The figure shows three views and two pictorial views of one solid part (mm, origin at its lowest corner). Answer the questions. A direction names the side the tool comes from. Coordinates: 2 decimals unless noted, no trailing zeros. Order: outer loops, then holes, each group sorted by start corner. A loop starts at its lowest first (then second) coordinate and runs counter-clockwise, first axis right, second up. Notation, with made-up numbers: M -26,66 L 24,66 A18 ccw 24,73 Z; hole C 9.5,48 d6. An arc over 180 degrees is marked long. Use a Markdown table: item, result.
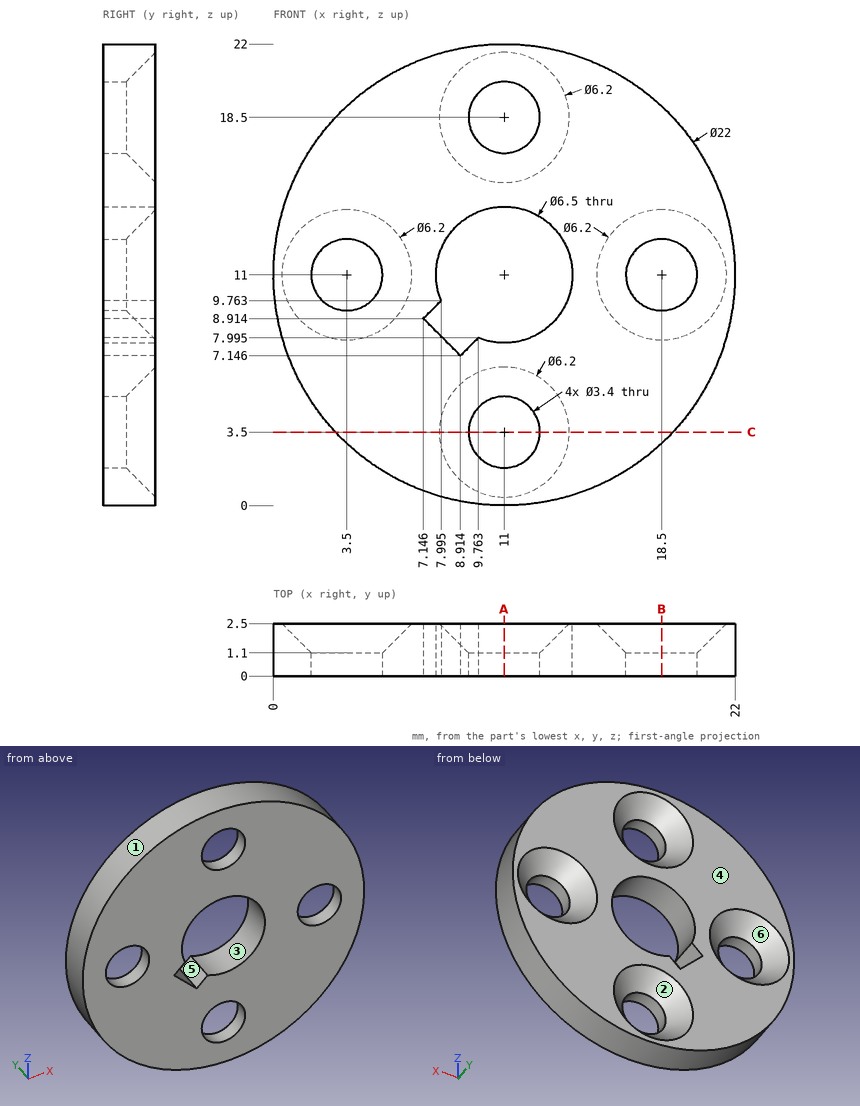
1. Section C-C on z = 3.5 is taken. Determine the outline of the cut face in (x, y).
Answers below:
| item | result |
|---|---|
| outline | M 2.95,0 L 9.3,0 L 9.3,1.1 L 7.9,2.5 L 2.95,2.5 Z; M 12.7,0 L 19.05,0 L 19.05,2.5 L 14.1,2.5 L 12.7,1.1 Z |
2. For a pull along Z with two mould halves and no side action, classify the marked faces 1, 2, 3 and 4 as +Z half, -Z half, draft (parallel to the pull), parting line (faces both ways), or undercut.
Answers below:
| item | result |
|---|---|
| face 1 | parting line |
| face 2 | undercut |
| face 3 | undercut |
| face 4 | draft |
3. Section B-B on x = 18.5 is taken. Determine the outline of the cut face in (y, z).
Answers below:
| item | result |
|---|---|
| outline | M 0,2.95 L 2.5,2.95 L 2.5,7.9 L 1.1,9.3 L 0,9.3 Z; M 0,12.7 L 1.1,12.7 L 2.5,14.1 L 2.5,19.05 L 0,19.05 Z |
4. Flat-ended cylindrical pins translate along their axes: P1, Ø4, axis at x = 11, z = 3.5, coming from the +Y side; P2, Ø2.5, axis at x = 18.5, z = 11, coming from the +Y side. Find the tip coordinate at first contact, or state that the pin passes through.
Answers below:
| item | result |
|---|---|
| P1 | y = 1.4 |
| P2 | through |
5. Find the intervals of material crossed by probe 1 along X at (y, z) = (0.7, 11); probe 2 along X at (y, z) = (1.6, 11.5) (1 decimal); probe 3 along Z at (x, y) = (8.75, 1.95) (1 decimal), in increasing order.
Answers below:
| item | result |
|---|---|
| probe 1 | 0 to 1.8, 5.2 to 7.75, 14.25 to 16.8, 20.2 to 22 |
| probe 2 | 0 to 1.4, 5.6 to 7.8, 14.2 to 16.4, 20.6 to 22 |
| probe 3 | 0.2 to 2.3, 4.7 to 7.3, 13.3 to 17.3, 19.7 to 21.8 |
6. Section A-A on x = 11 is taken. Determine the outline of the cut face in (y, z).
Answers below:
| item | result |
|---|---|
| outline | M 0,0 L 2.5,0 L 2.5,0.4 L 1.1,1.8 L 0,1.8 Z; M 0,5.2 L 1.1,5.2 L 2.5,6.6 L 2.5,7.75 L 0,7.75 Z; M 0,14.25 L 2.5,14.25 L 2.5,15.4 L 1.1,16.8 L 0,16.8 Z; M 0,20.2 L 1.1,20.2 L 2.5,21.6 L 2.5,22 L 0,22 Z |
7. For the marked faces 5 and 6, determine the directions among +Z, -Z, +X, -X, +Y, -Y from which every point of the face is accessible in a straight line to the end or side of a thin tool.
Answers below:
| item | result |
|---|---|
| face 5 | +Y, -Y |
| face 6 | +Y |
